Can you work these out from the model? Positions are in its coordinate system, mm. Face numbers are marked on the shaded views. A direction names the side the tool comes from. Give positions to 0.01 mm unless a question says otherwise; leave off trailing zeros. Write each loop counter-clockwise with the first axis right and the second up, starting at its lowest first coordinate (ties: lowest second). Pieces come first, ordered by that corner, then holes.
```python
from build123d import *

# Parameters (mm, degrees)
SKETCH1_R           = 15.875
SKETCH1_R_2         = 1.95
SKETCH1_R_3         = 6.35
BOSS_EXTRUDE1_DEPTH = 5.08
BOSS_EXTRUDE2_START = 6.35
SKETCH1_3_R         = 3.175
SKETCH1_3_R_2       = 1.95
BOSS_EXTRUDE2_DEPTH = 6.35
SKETCH2_R           = 15.875
SKETCH2_R_2         = 9.5
BOSS_EXTRUDE3_DEPTH = 6


with BuildPart() as part:
    # Sketch1 → Boss-Extrude1 (new body)
    with BuildSketch(Plane.XY):
        Circle(SKETCH1_R)
        with Locations((0, 12.7)):
            Circle(SKETCH1_R_2, mode=Mode.SUBTRACT)
        with Locations((0, -12.7)):
            Circle(SKETCH1_R_2, mode=Mode.SUBTRACT)
        Circle(SKETCH1_R_3, mode=Mode.SUBTRACT)
    extrude(amount=-BOSS_EXTRUDE1_DEPTH)

    # Sketch1_3 → Boss-Extrude2 (add)
    # profile 1 of 2: a face of its own
    with BuildSketch(Plane.XY.offset(BOSS_EXTRUDE2_START)):
        with Locations(Location((0, 12.7, 0), (0, 0, 89.999491584))):
            Circle(SKETCH1_3_R)
        with Locations((0, 12.7)):
            Circle(SKETCH1_3_R_2, mode=Mode.SUBTRACT)
    # profile 2 of 2: a face of its own
    with BuildSketch(Plane.XY.offset(BOSS_EXTRUDE2_START)):
        with Locations(Location((0, -12.7, 0), (0, 0, 269.999491584))):
            Circle(SKETCH1_3_R)
        with Locations((0, -12.7)):
            Circle(SKETCH1_3_R_2, mode=Mode.SUBTRACT)
    extrude(amount=-BOSS_EXTRUDE2_DEPTH)

    # Sketch2 → Boss-Extrude3 (add)
    with BuildSketch(Plane(origin=(0, 0, -5.08), x_dir=(-1, 0, 0), z_dir=(0, 0, -1))):
        with Locations(Location((0, 0, 0), (0, 0, 270))):
            Circle(SKETCH2_R)
        Circle(SKETCH2_R_2, mode=Mode.SUBTRACT)
    extrude(amount=BOSS_EXTRUDE3_DEPTH)


solid = part.part
```
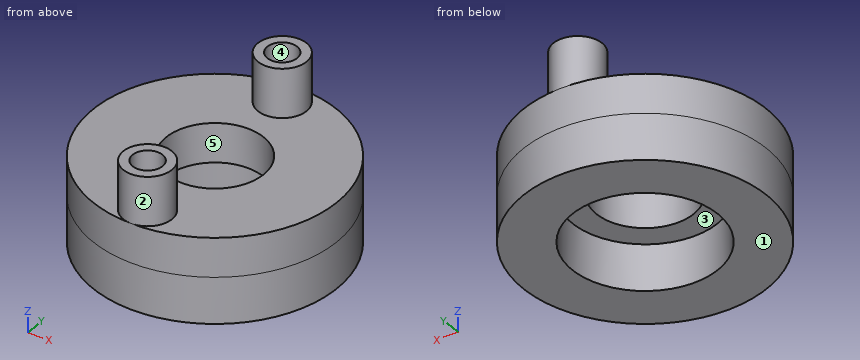
1) Suppose I cut it at B-B on x = -1. Write out the boundary of the cut face in (y, z), plus the area to 3 significant figures.
Values follow:
outline: (-15.84, -11.08) - (-9.45, -11.08) - (-9.45, -5.08) - (-6.27, -5.08) - (-6.27, 0) - (-9.69, 0) - (-9.69, 6.35) - (-11.03, 6.35) - (-11.03, -5.08) - (-14.37, -5.08) - (-14.37, 6.35) - (-15.71, 6.35) - (-15.71, 0) - (-15.84, 0) - close; (6.27, -5.08) - (9.45, -5.08) - (9.45, -11.08) - (15.84, -11.08) - (15.84, 0) - (15.71, 0) - (15.71, 6.35) - (14.37, 6.35) - (14.37, -5.08) - (11.03, -5.08) - (11.03, 6.35) - (9.69, 6.35) - (9.69, 0) - (6.27, 0) - close
area: 174 mm2
2) Suppose I cut it at D-D on x = 7.5. Write out the boundary of the cut face in (y, z), plus the area to 3 significant figures.
Values follow:
outline: (-13.99, -11.08) - (-5.83, -11.08) - (-5.83, -5.08) - (5.83, -5.08) - (5.83, -11.08) - (13.99, -11.08) - (13.99, 0) - (-13.99, 0) - close
area: 240 mm2
3) Suppose I cut it at A-A on y = 0. Write out the boundary of the cut face in (x, z) (3 decimals).
Values follow:
outline: (-15.875, -11.08) - (-9.5, -11.08) - (-9.5, -5.08) - (-6.35, -5.08) - (-6.35, 0) - (-15.875, 0) - close; (6.35, -5.08) - (9.5, -5.08) - (9.5, -11.08) - (15.875, -11.08) - (15.875, 0) - (6.35, 0) - close
4) If we mould it in two halves opening along Y, with no side actions, what happens to the marked faces 1 and 2? For each: +Y half, -Y half, draft (parallel to the pull), parting line (faces both ways), or undercut.
Values follow:
face 1: draft
face 2: undercut
5) For pin 1 Ø15 at (x, y) = (0, 0) entering from -Z; pin 2 Ø2 at (x, z) = (-11.5, -3.5) entering from +Y; pin 3 Ø1.5 at (x, z) = (12.5, -0.5) entering from +Y, each with a flat end and sliding along its axis, tell me the tip position at first contact or that it passes through.
Values follow:
pin 1: stops at z = -5.08
pin 2: stops at y = 11.91
pin 3: stops at y = 10.67
6) Suppose I cut it at C-C on y = -12.7. Write out the boundary of the cut face in (x, z) (3 decimals), plus the area to 3 significant figures.
Values follow:
outline: (-9.525, -11.08) - (9.525, -11.08) - (9.525, 0) - (3.175, 0) - (3.175, 6.35) - (1.95, 6.35) - (1.95, -5.08) - (-1.95, -5.08) - (-1.95, 6.35) - (-3.175, 6.35) - (-3.175, 0) - (-9.525, 0) - close
area: 207 mm2
7) Please list where these lines run through material, in increasing order: L1, parallel to Y at x = 0, z = -3.85 (3 decimals); L2, parallel to Y at x = 0, z = 0.75 (3 decimals); L3, parallel to X at y = -12.5, z = 1.
Values follow:
L1: y = -15.875 to -14.65, -10.75 to -6.35, 6.35 to 10.75, 14.65 to 15.875
L2: y = -15.875 to -14.65, -10.75 to -9.525, 9.525 to 10.75, 14.65 to 15.875
L3: x = -3.17 to -1.94, 1.94 to 3.17
8) For the marked faces 3, 4 and 5, which set-ups out of +Z, -Z, +X, -X, +Y, -Y let a thin tool reach every point of the face, with its end or its side?
Values follow:
face 3: -Z
face 4: +Z
face 5: +Z, -Z
